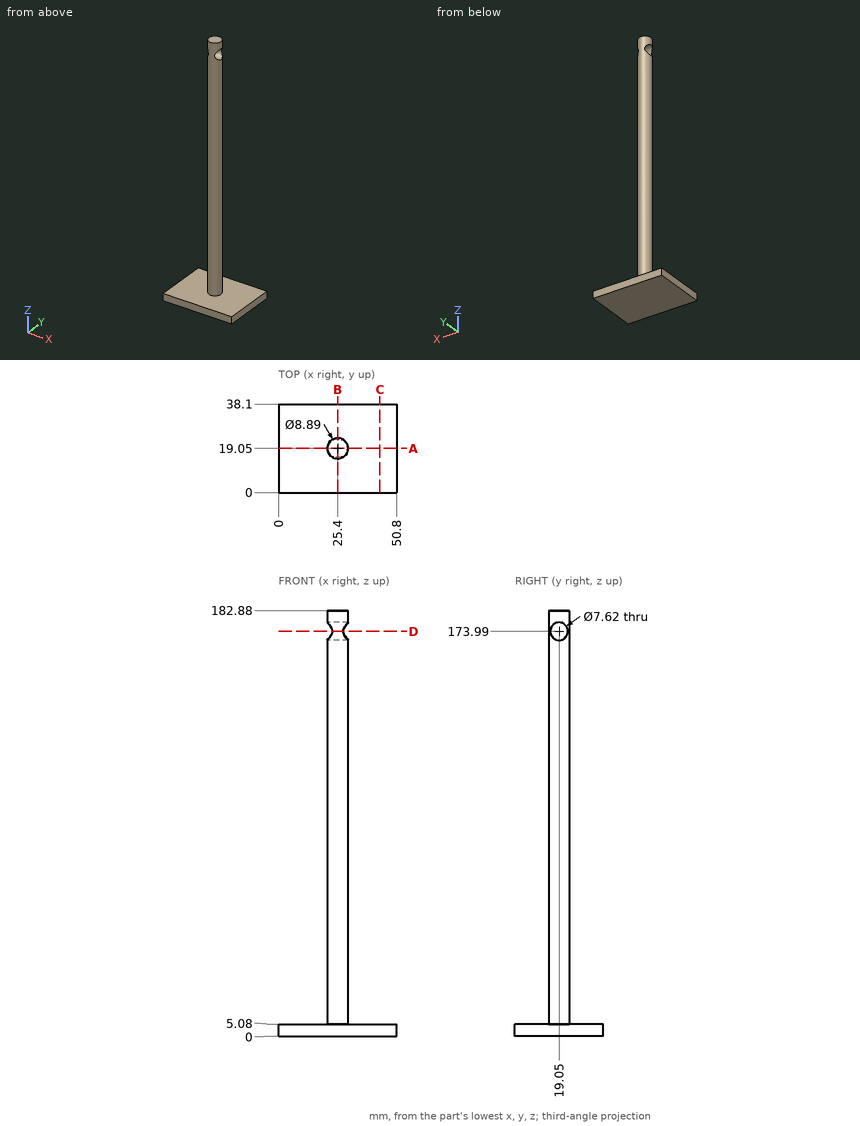
Study the drawing (mm; zero at the part's minimum x, y, z) and answer. Round coordinates to 2 decimals unless told otherwise and drop trailing zeros. Loops run counter-clockwise (first coordinate to the right, second up) from the corner with the lowest first, then second, coordinate; pieces in that order, holes last.
Q1. Section C-C, the plane x = 43.5 is taken. Determine the outline of the cut face in (y, z), then the cut area to 3 significant figures.
Q2. Find the intervals of material crossed by line 1 (Z direction, x = 27, y = 19); line 2 (Z direction, x = 20, y = 35); line 3 (Y direction, x = 27, z = 173), in increasing order.
Q3. Section D-D, the plane z = 173.99 is taken. Determine the outline of the cut face in (x, y) (3 decimals).
Q4. Section B-B, the plane x = 25.4 is taken. Determine the outline of the cut face in (y, z) (3 decimals), then the cut area to 3 significant figures.
Q5. Section A-A, the plane y = 19.05 is taken. Determine the outline of the cut face in (x, z) (3 decimals).
Q6. Given pin 1 Ø5 at (y, z) = (19.5, 40) entering from -X (3 decimals); pin 2 Ø12 at (y, z) = (19.05, 173.99) entering from +X (3 decimals); pin 3 Ø10 at (x, z) = (34, 20.5) entering from -Y, each flat-ended and moving along its own axis, determine where each tip first touches the part or whether it passes through.
Completed:
1. outline: (0, 0) - (38.1, 0) - (38.1, 5.08) - (0, 5.08) - close
1. area: 194 mm2
2. line 1: z = 0 to 170.18, 177.8 to 182.88
2. line 2: z = 0 to 5.08
2. line 3: y = 14.9 to 15.37, 22.73 to 23.2
3. outline: (23.11, 15.24) arc R4.445 ccw to (27.69, 15.24) - close; (23.11, 22.86) - (27.69, 22.86) arc R4.445 ccw to start
4. outline: (0, 0) - (38.1, 0) - (38.1, 5.08) - (23.495, 5.08) - (23.495, 182.88) - (14.605, 182.88) - (14.605, 5.08) - (0, 5.08) - close; hole circle Ø7.62 at (19.05, 173.99)
4. area: 1,730 mm2
5. outline: (0, 0) - (50.8, 0) - (50.8, 5.08) - (29.845, 5.08) - (29.845, 170.18) - (20.955, 170.18) - (20.955, 5.08) - (0, 5.08) - close; (20.955, 177.8) - (29.845, 177.8) - (29.845, 182.88) - (20.955, 182.88) - close
6. pin 1: stops at x = 20.955
6. pin 2: stops at x = 29.845
6. pin 3: stops at y = 16.44
